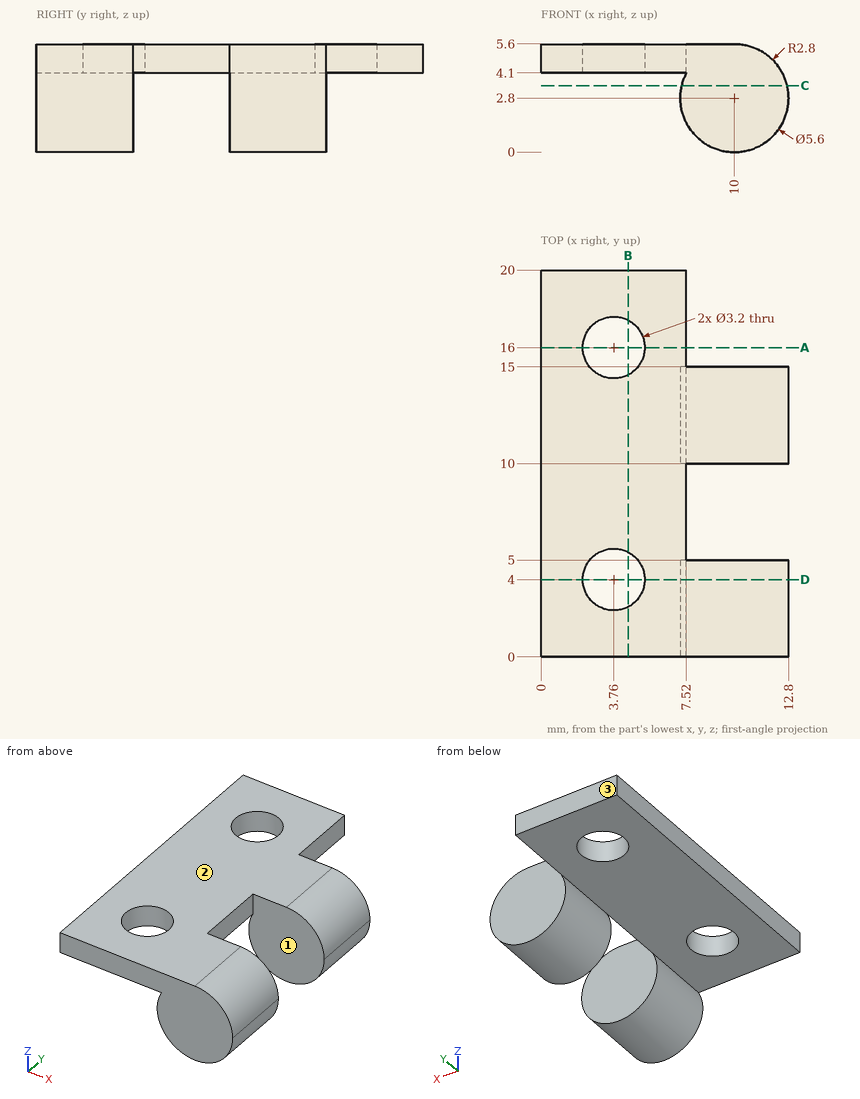
Study the drawing (mm; zero at the part's minimum x, y, z) and answer. Round coordinates to 2 decimals unless told otherwise and drop trailing zeros. Loops run counter-clockwise (first coordinate to the right, second up) from the corner with the lowest first, then second, coordinate; pieces in that order, holes last. Notation, with made-up numbers: (82, 81.25) -> (99, 81.25) arc R17 ccw to (99, 98.25) -> close; hole circle Ø9 at (57, 18). An arc over 180 degrees is marked (long way). One line per item, written item: value.
1) A cutting plane is placed at C-C (z = 3.45). Determine the outline of the cut face in (x, y).
Answer list:
outline: (7.28, 0) -> (12.72, 0) -> (12.72, 5) -> (7.28, 5) -> close; (7.28, 10) -> (12.72, 10) -> (12.72, 15) -> (7.28, 15) -> close
2) A cutting plane is placed at B-B (x = 4.5). Determine the outline of the cut face in (y, z), and give its area (3 significant figures).
Answer list:
outline: (0, 4.1) -> (2.58, 4.1) -> (2.58, 5.6) -> (0, 5.6) -> close; (5.42, 4.1) -> (14.58, 4.1) -> (14.58, 5.6) -> (5.42, 5.6) -> close; (17.42, 4.1) -> (20, 4.1) -> (20, 5.6) -> (17.42, 5.6) -> close
area: 21.5 mm²
3) A cutting plane is placed at A-A (y = 16). Determine the outline of the cut face in (x, z), and give its area (3 significant figures).
Answer list:
outline: (0, 4.1) -> (2.16, 4.1) -> (2.16, 5.6) -> (0, 5.6) -> close; (5.36, 4.1) -> (7.52, 4.1) -> (7.52, 5.6) -> (5.36, 5.6) -> close
area: 6.48 mm²
4) Consider L1, parallel to Y at x = 3, z = 4.95; L2, parallel to Y at x = 12, z = 3.3; L3, parallel to Z at x = 4.25, y = 12. Determine where each line is inside the solid, lowest interval first. Write a range as [from, to].
Answer list:
L1: y = [0, 2.59], [5.41, 14.59], [17.41, 20]
L2: y = [0, 5], [10, 15]
L3: z = [4.1, 5.6]
5) Flat-ended cylindrical pins translate along their axes: P1, Ø3, axis at x = 11.5, z = 1.5, coming from the +Y side; P2, Ø0.8, axis at y = 17.5, z = 5, coming from the +X side; P3, Ø1, axis at x = 6, y = 14, coming from the -Z side. Find the tip coordinate at first contact, or state that the pin passes through.
Answer list:
P1: stops at y = 15
P2: stops at x = 7.52
P3: stops at z = 4.1
6) A cutting plane is placed at D-D (y = 4). Determine the outline of the cut face in (x, z), and give its area (3 significant figures).
Answer list:
outline: (0, 4.1) -> (2.16, 4.1) -> (2.16, 5.6) -> (0, 5.6) -> close; (5.36, 4.1) -> (7.52, 4.1) arc R2.8 ccw (long way) to (10, 5.6) -> (5.36, 5.6) -> close
area: 32.2 mm²
7) The mould has two halves that part along Y. Classify the marked faces 1, 2 and 3: pulls with the +Y half, pulls with the -Y half, needs draft (parallel to the pull), parting line crosses it, or undercut.
Answer list:
face 1: undercut
face 2: needs draft
face 3: pulls with the +Y half
